The figure shows three views and two pictorial views of one solid part (mm, origin at its lowest corner). Answer the questions. A direction names the side the tool comes from. Give positions to 0.01 mm unless a question says otherwise; leave off trailing zeros. Loops run counter-clockwise (first coordinate to the right, second up) from the corner with the lowest first, then second, coordinate; pieces in that order, holes last. Notation, with made-up numbers: M -32.5,-34.5 L -4.5,-34.5 A8 ccw -4.5,-30.5 Z; hole C 77.5,-24 d3. An arc over 180 degrees is marked long. Write item = value, one per line. Start each with the question number.
1. Flat-ended cylindrical pins translate along their axes: pin 1 Ø2 at (x, z) = (10.5, 4) entering from +Y; pin 2 Ø10 at (y, z) = (34.5, 4) entering from -X; pin 3 Ø2 at (x, y) = (60.5, 53) entering from -Z; pin 4 Ø8 at (y, z) = (13.5, 4.5) entering from +X. Find the tip coordinate at first contact, or state that the pin passes through.
2. Section C-C on z = 14.5 is taken. Determine the outline of the cut face in (x, y) (3 decimals).
3. For the marked faces 1 and 2, determine the directions among +Z, -Z, +X, -X, +Y, -Y from which every point of the face is accessible in a straight line to the end or side of a thin tool.
4. Section A-A on x = 40 is taken. Determine the outline of the cut face in (y, z) (3 decimals), plus the area to 3 significant figures.
5. Consider L1, parallel to Z at x = 27, y = 57.5; L2, parallel to Y at x = 52.5, z = 7; L3, parallel to Y at x = 31, z = 9.25. Determine where each line is inside the solid, lowest interval first. Write a range as [from, to].
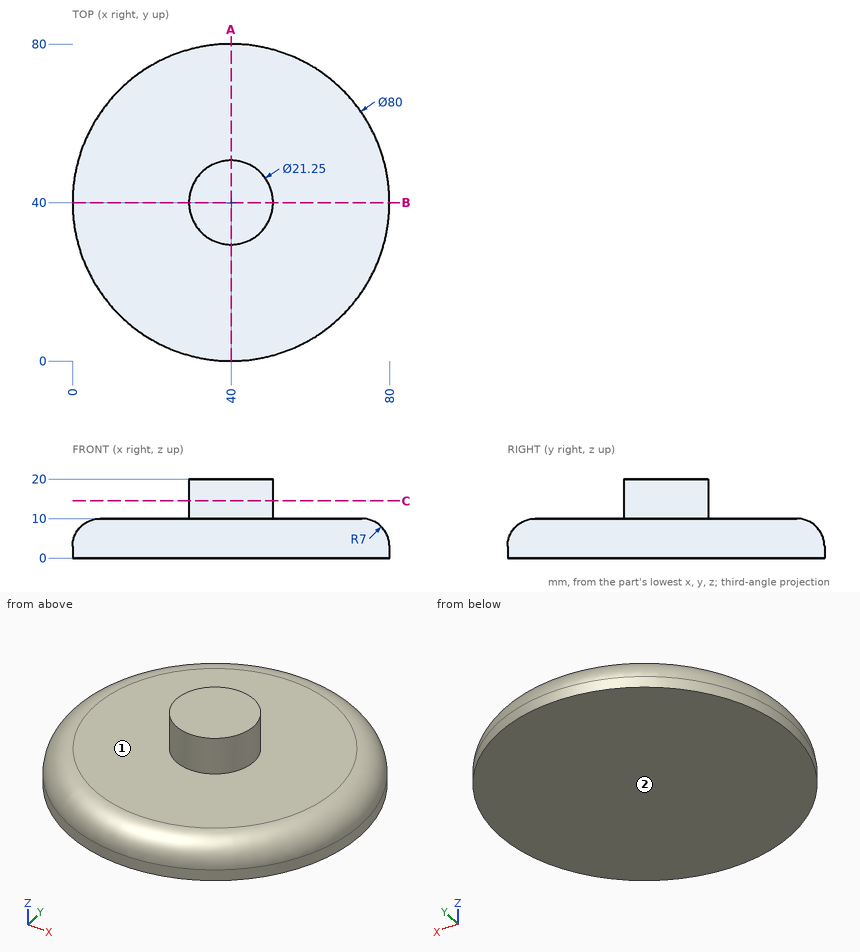
Verdict:
q1.pin_1 = 67.98
q1.pin_2 = 0
q1.pin_3 = 0
q1.pin_4 = 72.97
q2.outline = C 40,40 d21.25
q3.face_1 = +Z
q3.face_2 = -Z, +X, -X, +Y, -Y
q4.outline = M 0,0 L 80,0 L 80,3 A7 ccw 73,10 L 50.625,10 L 50.625,20 L 29.375,20 L 29.375,10 L 7,10 A7 ccw 0,3 Z
q4.area = 991 mm2
q5.L1 = [0, 10]
q5.L2 = [3.33, 76.67]
q5.L3 = [4.99, 75.01]
